Check sheet for the drawn part. Datum: minimum x, y, z corner. Units: mm. A direction names the side the tool comes from. Give positions to 0.01 mm unless a question says otherwise; leave off trailing zeros. Write each loop counter-clockwise with the first axis right and the second up, starting at its lowest first coordinate (ties: lowest second). Pieces come first, ordered by that corner, then holes. Notation, with made-up numbers: (-4.75, -38.5) - (7.25, -38.5) arc R34 ccw to (7.25, -7.5) - close; hole circle Ø7 at (46.25, 76.25). An arc over 180 degrees is marked (long way). Use a Markdown table: item, result.
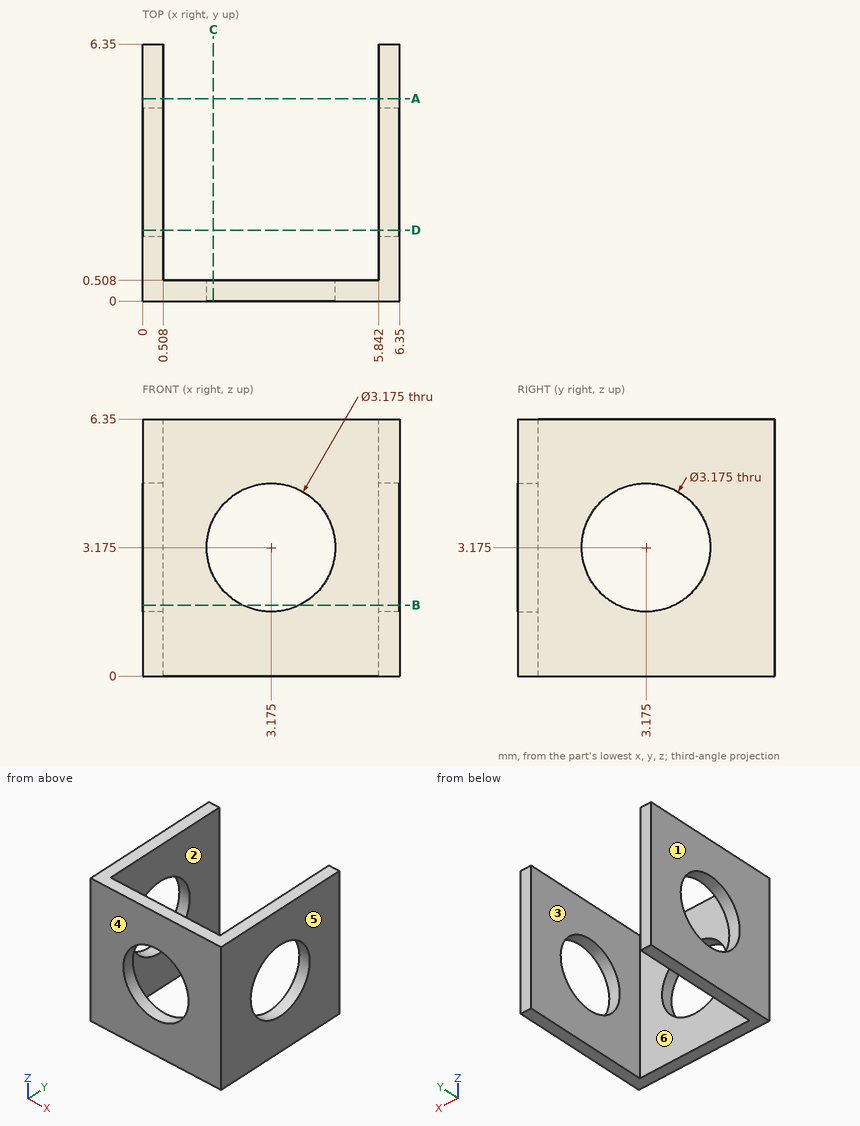
1) Depth check by flat-ended pin: P1, Ø1.5, axis at x = 4, z = 1.5, coming from the +Y side. Enter the tip coordinate at first touch or a pass-through.
Working result:
| item | result |
|---|---|
| P1 | stops at y = 0.51 |
2) Material ranges on L1, parallel to X at y = 3.75, z = 1.25; L2, parallel to Y at x = 0.75, z = 0.5, recorded low to high. Write a range as from..to.
Working result:
| item | result |
|---|---|
| L1 | x = 0..0.51, 5.84..6.35 |
| L2 | y = 0..0.51 |
3) Section check D-D on y = 1.75. Record the boundary of the cut face in (x, z).
Working result:
| item | result |
|---|---|
| outline | (0, 0) - (0.51, 0) - (0.51, 2.48) - (0, 2.48) - close; (0, 3.87) - (0.51, 3.87) - (0.51, 6.35) - (0, 6.35) - close; (5.84, 0) - (6.35, 0) - (6.35, 2.48) - (5.84, 2.48) - close; (5.84, 3.87) - (6.35, 3.87) - (6.35, 6.35) - (5.84, 6.35) - close |
4) Section check A-A on y = 5. Record the boundary of the cut face in (x, z).
Working result:
| item | result |
|---|---|
| outline | (0, 0) - (0.51, 0) - (0.51, 6.35) - (0, 6.35) - close; (5.84, 0) - (6.35, 0) - (6.35, 6.35) - (5.84, 6.35) - close |
5) Section check B-B on z = 1.75. Record the boundary of the cut face in (x, y).
Working result:
| item | result |
|---|---|
| outline | (0, 0) - (2.48, 0) - (2.48, 0.51) - (0.51, 0.51) - (0.51, 2.48) - (0, 2.48) - close; (0, 3.87) - (0.51, 3.87) - (0.51, 6.35) - (0, 6.35) - close; (3.87, 0) - (6.35, 0) - (6.35, 2.48) - (5.84, 2.48) - (5.84, 0.51) - (3.87, 0.51) - close; (5.84, 3.87) - (6.35, 3.87) - (6.35, 6.35) - (5.84, 6.35) - close |
6) Mould release check, pull along X, two halves, no side actions. Record for the marked faces 1, 2, 3 and 4: pulls with the +X half, pulls with the -X half, needs draft (parallel to the pull), parting line crosses it, or undercut.
Working result:
| item | result |
|---|---|
| face 1 | pulls with the -X half |
| face 2 | undercut |
| face 3 | undercut |
| face 4 | needs draft |
7) Set-up check for the marked faces 5 and 6: record each of +Z, -Z, +X, -X, +Y, -Y from which the full face is reachable in a straight line by a thin tool's end or side.
Working result:
| item | result |
|---|---|
| face 5 | +Z, -Z, +X, +Y, -Y |
| face 6 | +Z, -Z, +Y |
8) Section check C-C on x = 1.75. Record the boundary of the cut face in (y, z).
Working result:
| item | result |
|---|---|
| outline | (0, 0) - (0.51, 0) - (0.51, 2.48) - (0, 2.48) - close; (0, 3.87) - (0.51, 3.87) - (0.51, 6.35) - (0, 6.35) - close |
